For this review, take the finished solid that the model builds, in its own axes (mm). Round coordinates to 2 decimals unless told otherwise and drop trailing zeros. Order: outer loops, then holes, each group sorted by start corner. A loop starts at its lowest first (then second) coordinate and runs counter-clockwise, first axis right, second up. Notation, with made-up numbers: (30, 7.25) - (67, 7.25) arc R24 ccw to (67, 18.25) - close; hole circle Ø6 at (88, 72). An arc over 180 degrees is marked (long way). One line per item, written item: value.
```python
from build123d import *

# Parameters (mm, degrees)
F0_W     = 20
F0_H     = 12.774734
F0_R     = 1.75
F0_R_2   = 1.181266
F0_H_2   = 17.225266
F0_R_3   = 1.079972
F0_R_4   = 0.05
F0_R_5   = 1.186285
F0_R_6   = 0.980798
F1_DEPTH = 1


with BuildPart() as f1:
    # F0 (on Front) → F1 (new body)
    with BuildSketch(Plane.XZ):
        with Locations((-10, 6.387367)):
            Rectangle(F0_W, F0_H)
        with Locations((-16.25, 9.024734)):
            Circle(F0_R, mode=Mode.SUBTRACT)
        with Locations((10, 6.387367)):
            Rectangle(F0_W, F0_H)
        with Locations((5.371809, 4.774734)):
            Circle(F0_R_2, mode=Mode.SUBTRACT)
        with Locations((-10, -8.612633)):
            Rectangle(F0_W, F0_H_2)
        with Locations((-16.25, -13.475266)):
            Circle(F0_R, mode=Mode.SUBTRACT)
        with Locations((-12, -2.225266)):
            Circle(F0_R_3, mode=Mode.SUBTRACT)
        Polygon((73, 12.774734), (20, 12.774734), (20, 0), (20, -17.225266), (73, -17.225266), align=None)
        with Locations((69.25, -13.475266)):
            Circle(F0_R, mode=Mode.SUBTRACT)
        with Locations((63, -2.225266)):
            Circle(F0_R_4, mode=Mode.SUBTRACT)
        with Locations((65, -2.225266)):
            Circle(F0_R_5, mode=Mode.SUBTRACT)
        with Locations((69.25, 9.024734)):
            Circle(F0_R, mode=Mode.SUBTRACT)
        with Locations((10, -8.612633)):
            Rectangle(F0_W, F0_H_2)
        with Locations((5.371809, -16.225266)):
            Circle(F0_R_6, mode=Mode.SUBTRACT)
    extrude(amount=F1_DEPTH)


solid = f1.part
```
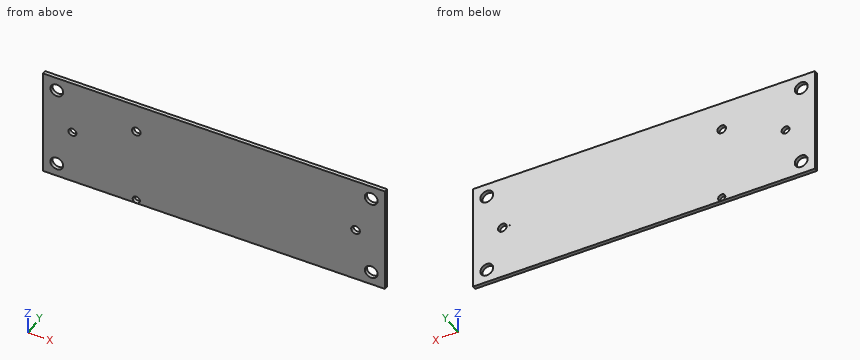
Item 1: Wall thickness on line 1 (Z direction, x = 69.25, y = -0.2); line 2 (X direction, y = -0.9, z = -1.75); line 3 (X direction, y = -0.3, z = 10.5): over which ranges is each line inside the solid? List them lowest first.
Returned:
line 1: -17.23 to -15.23, -11.73 to 7.27, 10.77 to 12.77
line 2: -20 to -12.97, -11.03 to 63.91, 66.09 to 73
line 3: -20 to -17.19, -15.31 to 68.31, 70.19 to 73
Item 2: For P1, Ø8, axis at x = 15.5, z = 3.5, coming from the +Y side; P2, Ø1.8, axis at x = 5.37, z = -16.23, coming from the -Y side, all flat-tipped, find the tip position at first contact; note any pin that passes through.
Returned:
P1: y = 0
P2: through
Item 3: Take a section at B-B (y = -0.5). Count the separate pieces of the cut face and the enclosed holes in it, plus the area to 3 significant figures.
Returned:
separate pieces: 1
enclosed holes: 9
area: 2,740 mm^2
Item 4: Take a section at A-A (x = 69.25). Write out the cut boundary in (y, z).
Returned:
outline: (-1, -17.23) - (0, -17.23) - (0, -15.23) - (-1, -15.23) - close; (-1, -11.73) - (0, -11.73) - (0, 7.27) - (-1, 7.27) - close; (-1, 10.77) - (0, 10.77) - (0, 12.77) - (-1, 12.77) - close
